from build123d import *

# Parameters (mm, degrees)
SKETCH_2_W             = 70
SKETCH_2_H             = 44
SM_BASE_FLANGE_1_DEPTH = 1.2
CUT_EXTRUDE_1_DEPTH    = 42.357466073
SKETCH_6_R             = 0.95
CUT_EXTRUDE_2_DEPTH    = 42.357466073


# Sheet-metal steps are written as plain solids
with BuildPart() as part:
    # 草图2 → 基体-法兰1 (new body)
    with BuildSketch(Plane.XY):
        Rectangle(SKETCH_2_W, SKETCH_2_H)
    extrude(amount=-SM_BASE_FLANGE_1_DEPTH)

    # 草图5 → 切除-拉伸1 (cut, through all)
    with BuildSketch(Plane.XY):
        with BuildLine():
            Line((39, -14), (35, -14))
            Line((35, -14), (35, -18))
            ThreePointArc((35, -18), (33.828427125, -15.171572875), (31, -14))
            Line((31, -14), (31, 14))
            ThreePointArc((31, 14), (33.828427125, 15.171572875), (35, 18))
            Line((35, 18), (35, 14))
            Line((35, 14), (39, 14))
            Line((39, 14), (39, -14))
        make_face()
        with BuildLine():
            Line((-39, -14), (-39, 14))
            Line((-39, 14), (-35, 14))
            Line((-35, 14), (-35, 18))
            ThreePointArc((-35, 18), (-33.828427125, 15.171572875), (-31, 14))
            Line((-31, 14), (-31, -14))
            ThreePointArc((-31, -14), (-33.828427125, -15.171572875), (-35, -18))
            Line((-35, -18), (-35, -14))
            Line((-35, -14), (-39, -14))
        make_face()
    extrude(amount=-CUT_EXTRUDE_1_DEPTH, mode=Mode.SUBTRACT)

    # 草图6 → 切除-拉伸2 (cut, through all)
    with BuildSketch(Plane.XY):
        with Locations((-10.153838394, 4.949747468)):
            Circle(SKETCH_6_R)
        with Locations((-0.254343457, 4.949747468)):
            Circle(SKETCH_6_R)
        with Locations((-0.254343457, -4.949747468)):
            Circle(SKETCH_6_R)
        with Locations((-10.153838394, -4.949747468)):
            Circle(SKETCH_6_R)
    extrude(amount=-CUT_EXTRUDE_2_DEPTH, mode=Mode.SUBTRACT)


solid = part.part
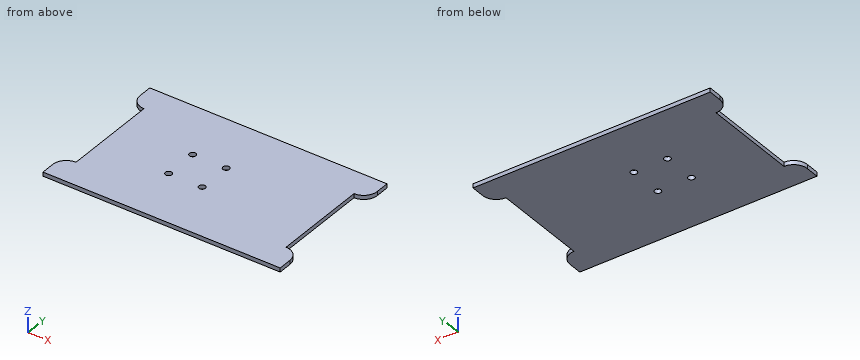
Check sheet for the modelled part. Datum: model origin and axes. Units: mm. Coordinates: 2 decimals unless noted, no trailing zeros. Write each loop counter-clockwise with the first axis right and the second up, starting at its lowest first coordinate (ties: lowest second). Pieces come first, ordered by that corner, then holes. Notation, with made-up numbers: M 12,74.25 L 48,74.25 A34 cw 48,112.25 Z; hole C -31,-25 d3. An arc over 180 degrees is marked long. Answer as CSV lines item,"result".
Q1. Cross-section at A-A (z = -0.55). Record the boundary of the cut face in (x, y).
Check result:
outline,"M -35,-22 L 35,-22 L 35,-18 A4 ccw 31,-14 L 31,14 A4 ccw 35,18 L 35,22 L -35,22 L -35,18 A4 ccw -31,14 L -31,-14 A4 ccw -35,-18 Z; hole C -10.15,-4.95 d1.9; hole C -10.15,4.95 d1.9; hole C -0.25,-4.95 d1.9; hole C -0.25,4.95 d1.9"
Q2. Material ranges on probe 1 along X at (y, z) = (7, -0.4); probe 2 along X at (y, z) = (-5.5, -0.3); probe 3 along X at (y, z) = (-17, -0.65), recorded low to high. Write a range as from..to.
Check result:
probe 1,"-31..31"
probe 2,"-31..-10.93, -9.38..-1.03, 0.52..31"
probe 3,"-34.87..34.87"
Q3. Go/stop test with flat-tipped pins: pin 1 (1.5 mm diameter, centred on x = -0.25, y = -4.95, fed in from -Z); pin 2 (0.6 mm diameter, centred on y = -4.5, z = -0.5, fed in from -X). Record where each tip stops, or that it passes through.
Check result:
pin 1,"through"
pin 2,"x = -31"
Q4. Cross-section at B-B (y = -8). Record the boundary of the cut face in (x, z).
Check result:
outline,"M -31,-1.2 L 31,-1.2 L 31,0 L -31,0 Z"
